Autodesk Inventor part; units mm, degrees
ref_plane "YZ Ebene" through (0, 0, 0) normal (1, 0, 0) x (0, 1, 0)
ref_plane "XZ Ebene" through (0, 0, 0) normal (0, 1, 0) x (-1, 0, 0)
ref_plane "XY Ebene" through (0, 0, 0) normal (0, 0, 1) x (1, 0, 0)
sketch "Sketch20" plane through (0, 0, 0) normal (0, 1, 0) x (-1, 0, 0)
  line L0 (0, 0) -> (120, 0)
  line L1 (120, 0) -> (120, -120)
  line L2 (120, -120) -> (0, -120)
  line L3 (0, -120) -> (0, 0)
  dimension "d58" = 120
  dimension "d59" = 120
extrude "Extrusion8" add sketch "Sketch20" against normal blind 5
fillet "Fillet5" radius 2 8 edges at (-60, -5, 0) (0, -2.5, 0) (0, -5, -60) (0, -2.5, -120) (-60, -5, -120) (-120, -5, -60) (-120, -2.5, -120) (-120, -2.5, 0)
sketch "Sketch21" plane through (0, -5, 0) normal (0, -1, 0) x (1, 0, 0)
  line L0 (-2, 0) -> (-118, 0)
  line L1 (0, -118) -> (0, -2)
  line L2 (-120, -2) -> (-120, -118)
  line L3 (-118, -120) -> (-2, -120)
  point P0 (0, 0)
  point P1 (-5, -5)
  point P2 (-60, -5)
  point P3 (-115, -5)
  point P4 (-115, -5)
  point P5 (-115, -115)
  point P6 (-5, -115)
  point P7 (-5, -60)
  point P8 (-115, -60)
  point P9 (-60, -115)
  dimension "d63" = 5
  dimension "d64" = 5
  dimension "d65" = 55
  dimension "d66" = 5
  dimension "d67" = 5
  dimension "d68" = 55
  dimension "d69" = 5
  dimension "d70" = 5
  dimension "d71" = 55
hole "Hole2" at (-5, -5, -5) at (-60, -5, -5) at (-115, -5, -5) at (-115, -5, -115) at (-5, -5, -115) at (-5, -5, -60) at (-115, -5, -60) at (-60, -5, -115) direction (0, 1, 0) diameter 2.46 depth 8.8 counterbore diameter 4 counterbore depth 2
properties part number "raspberry_box_lid" material "S235JR"
Could you check a few things on this model? Use its own coordinates, in mm. A direction names the side the tool comes from. Give positions to 0.01 mm unless a question says otherwise; leave off trailing zeros. Return JSON: item names as keys, results as strings.
Item 1: I need wall thicknesses on L1, parallel to Z at x = -115, y = -1.6; L2, parallel to Z at x = -60, y = -1.3. Which ranges of each line are inside material? Lowest first, please. Write a range as from..to.
Geometry results:
{"L1": "z = -120..-116.23, -113.77..-61.23, -58.77..-6.23, -3.77..0", "L2": "z = -120..-116.23, -113.77..-6.23, -3.77..0"}
Item 2: I'm going to push flat-ended pins straight in: pin 1 (3 mm diameter, centred on x = -115, z = -115, fed in from +Y); pin 2 (2 mm diameter, centred on x = -60.5, z = -5, fed in from -Y). Where does each tip first touch, or does it pass through?
Geometry results:
{"pin 1": "stops at y = 0", "pin 2": "stops at y = -3"}
Item 3: Which directions (+Z, -Z, +X, -X, +Y, -Y) give clear straight access to the entire face, cutting with the end or side of a thin tool? Please do faces 1 (the flat face through (0, -1, -61)), 2 (the flat face through (-4, -3, -59)).
Geometry results:
{"face 1": "+Z, -Z, +X, +Y, -Y", "face 2": "-Y"}
Item 4: We'd pull the mould along Z, two halves only. Please class faces 3 (the flat face through (-4, -3, -4)), 4 (the flat face through (-120, -1, -59)), 5 (the flat face through (-61, -1, -120)): +Z half, -Z half, draft (parallel to the pull), parting line (faces both ways), or undercut.
Geometry results:
{"face 3": "undercut", "face 4": "draft", "face 5": "-Z half"}
